Autodesk Inventor part; units mm, degrees
ref_plane "YZ Plane" through (0, 0, 0) normal (1, 0, 0) x (0, 1, 0)
ref_plane "XZ Plane" through (0, 0, 0) normal (0, 1, 0) x (-1, 0, 0)
ref_plane "XY Plane" through (0, 0, 0) normal (0, 0, 1) x (1, 0, 0)
ref_plane "Work Plane1" through (0, 0, 0) normal (0, 0, 1) x (1, 0, 0)
sketch "Sketch1" plane through (0, 0, 0) normal (0, 0, 1) x (1, 0, 0)
  circle A0 centre (64.078, -33.7875) radius 2.5
  circle A1 centre (113.8201, -38.8599) radius 2.5
  circle A2 centre (108.7476, 10.8821) radius 2.5
  circle A3 centre (91.0159, -16.0557) radius 21.5
  circle A4 centre (136.9222, 103.1056) radius 10
  circle A5 centre (-113.0778, -14.3944) radius 27.5
  circle A6 centre (-124.7161, 93.1056) radius 31
  circle A7 centre (111.9222, 55.1056) radius 15
  arc A8 (-163.0778, -77.8944) -> (-203.0778, -77.8944) centre (-183.0778, -73.3944) ccw
  line L0 (-203.0778, -77.8944) -> (-163.0778, -77.8944)
  circle A9 centre (4.8797, -98.3944) radius 10
  circle A10 centre (36.9222, 38.038) radius 29
  line L1 (-105.1203, -129.3944) -> (114.8797, -129.3944)
  line L2 (114.8797, -129.3944) -> (245.5334, -114.7214)
  line L3 (245.5334, -114.7214) -> (212.3797, 137.1056)
  line L4 (212.3797, 137.1056) -> (-202.6203, 137.1056)
  line L5 (-202.6203, 137.1056) -> (-249.3685, -103.3931)
  line L6 (-249.3685, -103.3931) -> (-206.3685, -103.3931)
  arc A11 (-204.3685, -105.3931) -> (-206.3685, -103.3931) centre (-206.3685, -105.3931) ccw
  line L7 (-204.3685, -105.3931) -> (-204.3685, -121.3931)
  line L8 (-204.3685, -121.3931) -> (-107.1203, -121.3931)
  arc A12 (-105.1203, -123.3931) -> (-107.1203, -121.3931) centre (-107.1203, -123.3931) ccw
  line L9 (-105.1203, -123.3931) -> (-105.1203, -129.3944)
  point P0 (0, 0)
extrude "Extrusion1" add sketch "Sketch1" along normal blind 25.4
sketch "Sketch2" plane through (0, 0, 25.4) normal (0, 0, 1) x (1, 0, 0)
  circle A0 centre (-184.4709, 24.8028) radius 22.2192
  point P0 (0, 0)
  dimension "Hole" = 44.4384
extrude "Extrusion2" cut sketch "Sketch2" against normal through all
properties part number "Part11.ipt-01"
The model under review builds one solid part; all positions refer to its coordinate system, in mm. A direction names the side the tool comes from. Give positions to 0.01 mm unless a question says otherwise; leave off trailing zeros. Write each loop counter-clockwise with the first axis right and the second up, starting at its lowest first coordinate (ties: lowest second). Pieces come first, ordered by that corner, then holes. Notation, with made-up numbers: M -31,47 L -20,47 A35 ccw -20,85 Z; hole C 34,52.5 d1. An arc over 180 degrees is marked long. One line per question, with ' | ' between items. Start each with the question number.
Item 1: For faces 4 (the flat face through (-204.368, -113, 13)), 5 (the flat face through (-5, 6, 0)), list the 3-axis set-ups (+Z, -Z, +X, -X, +Y, -Y) from which the entire face can be reached by the end or side of a thin tool; tool diameter is ignored.
Item 2: Wall thickness on line 1 (X direction, y = 37.5, z = 3); line 2 (Y direction, x = 104.5, z = 17); line 3 (X direction, y = -22, z = 3): over which ranges is each line inside the solid? List them lowest first. Write a range as from..to.
Item 3: We need section D-D on x = 173. Write out the cut boundary in (y, z).
Item 4: We need section A-A on x = -151. Write out the cut boundary in (y, z).
Item 5: Draft analysis for pull direction X (two halves, no side actions). For faces 1 (the flat face through (8, 137.106, 13)), 2 (the cylindrical face through (7.95, 36.76, 12.52)), 3 (the flat face through (179.29, -122.16, 12.52)), state which applies: released by +X, released by -X, zero draft, split by the parting line, or undercut.
Item 6: We need section C-C on z = 18. Give the number of separate pieces and of enclosed holes in the cut face, plus the area to 3 significant figures.
Item 7: For pin 1 (12.5 mm diameter, centred on x = -157, z = 16, fed in from -Y); pin 2 (1.5 mm diameter, centred on y = -64, z = 6.5, fed in from +X); pin 3 (18 mm diameter, centred on x = 4.88, y = -98.39, fed in from +Z); pin 4 (1 mm diameter, centred on y = 63.5, z = 13, fed in from -X), all flat-tipped, find the tip position at first contact; note any pin that passes through.
Item 8: We need section B-B on y = -6. Write out the cut boundary in (x, z).
Results found:
1) face 4: +Z, -Z, -X, -Y | face 5: -Z, +X, -X, +Y, -Y
2) line 1: x = -221.98..-202.7, -166.24..7.93, 65.92..225.49 | line 2: y = -129.39..-32.8, 0.69..42.07, 68.14..137.11 | line 3: x = -233.55..-139.51, -86.65..70.35, 111.68..233.33
3) outline: M -122.87,0 L 137.11,0 L 137.11,25.4 L -122.87,25.4 Z
4) outline: M -121.39,0 L 76.67,0 L 76.67,25.4 L -121.39,25.4 Z; M 109.54,0 L 137.11,0 L 137.11,25.4 L 109.54,25.4 Z
5) face 1: zero draft | face 2: undercut | face 3: released by +X
6) separate pieces: 1 | enclosed holes: 12 | area: 106,000 mm2
7) pin 1: stops at y = -121.39 | pin 2: stops at x = 238.95 | pin 3: passes through | pin 4: stops at x = -217.02
8) outline: M -230.44,0 L -139.27,0 L -139.27,25.4 L -230.44,25.4 Z; M -86.89,0 L 72.01,0 L 72.01,25.4 L -86.89,25.4 Z; M 110.02,0 L 231.22,0 L 231.22,25.4 L 110.02,25.4 Z
